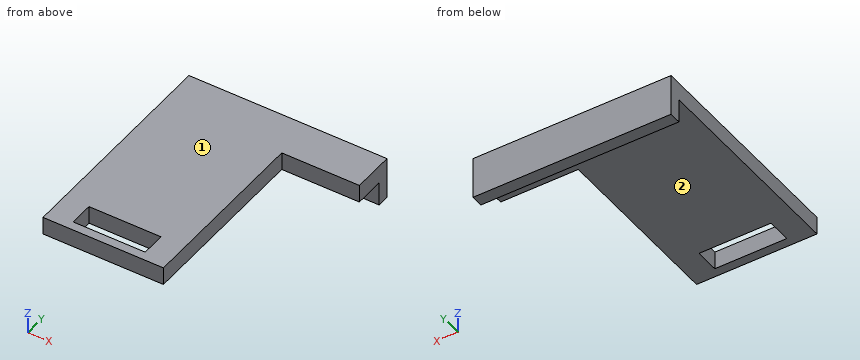
Autodesk Inventor part; units mm, degrees
ref_plane "YZ Plane" through (0, 0, 0) normal (1, 0, 0) x (0, 1, 0)
ref_plane "XZ Plane" through (0, 0, 0) normal (0, 1, 0) x (-1, 0, 0)
ref_plane "XY Plane" through (0, 0, 0) normal (0, 0, 1) x (1, 0, 0)
sketch "Sketch1" plane through (0, 0, 0) normal (0, 0, 1) x (1, 0, 0)
  line L0 (-3.1754, 5) -> (-49.0181, 5)
  line L1 (-3.1754, 40) -> (-3.1754, 5)
  line L2 (-97.8609, 40) -> (-3.1754, 40)
  line L3 (-97.8609, 5) -> (-97.8609, 40)
  line L4 (-52.0181, 5) -> (-97.8609, 5)
  line L5 (-52.0181, 5) -> (-52.0181, 37)
  line L6 (-52.0181, 37) -> (-49.0181, 37)
  line L7 (-49.0181, 37) -> (-49.0181, 5)
  line L8 (-52.0181, 5) -> (-85.0042, 5)
  line L9 (-85.0042, 5) -> (-85.0042, 50)
  line L10 (-85.0042, 50) -> (-52.0181, 50)
  line L11 (-52.0181, 50) -> (-52.0181, 5)
  line L12 (-52.0181, 10.5351) -> (-74.9481, 10.5351) construction
  point P0 (0, 0)
  point P1 (-66.8598, 10.5351)
  dimension "d1" = 45
  dimension "d7" = 45.8427
  dimension "d8" = 22.93
extrude "Extrusion1" add sketch "Sketch1" along normal blind 3 contours L11 L5 L4 L9 L2 | L2 L9 L10 L11
sketch "Sketch2" plane through (0, 0, 0) normal (0, 0, -1) x (-1, 0, 0)
  line L0 (95.2628, 40) -> (95.2628, 0)
  line L1 (5.7735, 40) -> (95.2628, 40)
  line L2 (5.7735, 0) -> (5.7735, 40)
  line L3 (95.2628, 0) -> (5.7735, 0)
  line L4 (52.0181, 5) -> (52.0181, 50)
  line L5 (85.0042, 5) -> (52.0181, 5)
  line L6 (85.0042, 50) -> (85.0042, 5)
  line L7 (52.0181, 50) -> (85.0042, 50)
  line L8 (52.0181, 50) -> (85.0042, 50)
  line L9 (85.0042, 50) -> (85.0042, 40)
  line L10 (85.0042, 40) -> (52.0181, 40)
  line L11 (52.0181, 40) -> (52.0181, 50)
  point P0 (0, 0)
extrude "Extrusion2" add sketch "Sketch2" along normal blind 4 contours L1 L4 L7 L6
sketch "Sketch3" plane through (0, 0, 3) normal (0, 0, 1) x (1, 0, 0)
  line L0 (-80.9481, 10.4777) -> (-68.9481, 10.4777)
  line L1 (-68.9481, 10.4777) -> (-68.9481, 6.4777)
  line L2 (-68.9481, 6.4777) -> (-80.9481, 6.4777)
  line L3 (-80.9481, 6.4777) -> (-80.9481, 10.4777)
  line L4 (-80.9481, 10.4777) -> (-68.9481, 6.4777) construction
  line L5 (-68.9481, 10.4777) -> (-80.9481, 6.4777) construction
  circle A0 centre (-74.9481, 8.4777) radius 2 construction
  circle A1 centre (-71.4481, 8.4777) radius 2 construction
  circle A2 centre (-71.7614, 8.4777) radius 2 construction
  line L6 (-52.0181, 5) -> (-52.0181, 50)
  point P0 (0, 0)
  point P1 (-71.4481, 8.4777)
  dimension "d9" = 12
  dimension "d10" = 4
  dimension "d11" = 4
  dimension "d12" = 3.5
  dimension "d13" = 3.5
  dimension "d23" = 22.93
extrude "Extrusion3" cut sketch "Sketch3" against normal blind 4
sketch "Sketch5" plane through (0, 0, 3) normal (0, 0, 1) x (1, 0, 0)
  line L0 (-80.9481, 6.4777) -> (-80.9481, 10.4777)
  line L1 (-80.9481, 10.4777) -> (-68.9481, 10.4777)
  line L2 (-68.9481, 10.4777) -> (-68.9481, 6.4777)
  line L3 (-68.9481, 6.4777) -> (-80.9481, 6.4777)
  line L4 (-52.0181, 5) -> (-52.0181, 50)
  line L5 (-52.0181, 50) -> (-85.0042, 50)
  line L6 (-85.0042, 50) -> (-85.0042, 5)
  line L7 (-85.0042, 5) -> (-52.0181, 5)
  line L8 (-64.9481, 5) -> (-64.9481, 35)
  line L9 (-64.9481, 35) -> (-52.0181, 35)
  point P0 (0, 0)
  dimension "d39" = 30
  dimension "d40" = 4
extrude "Extrusion5" cut sketch "Sketch5" against normal blind 4 contours L7 L8 L9 L4
chamfer "Chamfer1" [suppressed]
sketch "Sketch6" plane through (0, 0, 3) normal (0, 0, 1) x (1, 0, 0)
  line L0 (-64.9481, 35) -> (-52.0181, 35)
  line L1 (-52.0181, 35) -> (-52.0181, 50)
  line L2 (-52.0181, 50) -> (-85.0042, 50)
  line L3 (-85.0042, 50) -> (-85.0042, 5)
  line L4 (-85.0042, 5) -> (-64.9481, 5)
  line L5 (-64.9481, 5) -> (-64.9481, 35)
  line L6 (-80.9481, 6.4777) -> (-80.9481, 10.4777)
  line L7 (-80.9481, 10.4777) -> (-68.9481, 10.4777)
  line L8 (-68.9481, 10.4777) -> (-68.9481, 6.4777)
  line L9 (-68.9481, 6.4777) -> (-80.9481, 6.4777)
  line L10 (-52.0181, 35) -> (-52.0181, 50)
  line L11 (-85.0042, 50) -> (-52.0181, 50)
  line L12 (-52.0181, 50) -> (-52.0181, 42)
  line L13 (-52.0181, 42) -> (-85.0042, 42)
  line L14 (-85.0042, 42) -> (-85.0042, 50)
  point P0 (0, 0)
  dimension "d44" = 8
extrude "Extrusion6" cut sketch "Sketch6" against normal blind 12.5 contours L13 L3 L2 L1
sketch "Sketch4" plane through (0, 0, 3) normal (0, 0, 1) x (1, 0, 0)
  line L0 (-80.9481, 6.4777) -> (-80.9481, 10.4777)
  line L1 (-80.9481, 10.4777) -> (-68.9481, 10.4777)
  line L2 (-68.9481, 10.4777) -> (-68.9481, 6.4777)
  line L3 (-68.9481, 6.4777) -> (-80.9481, 6.4777)
  line L4 (-52.0181, 5) -> (-52.0181, 50)
  line L5 (-52.0181, 50) -> (-85.0042, 50)
  line L6 (-85.0042, 50) -> (-85.0042, 5)
  line L7 (-85.0042, 5) -> (-52.0181, 5)
  line L8 (-81.0042, 47) -> (-56.0181, 47)
  line L9 (-56.0181, 47) -> (-56.0181, 42)
  line L10 (-56.0181, 42) -> (-81.0042, 42)
  line L11 (-81.0042, 42) -> (-81.0042, 47)
  line L12 (-81.0042, 38) -> (-56.0181, 38)
  line L13 (-56.0181, 38) -> (-56.0181, 33)
  line L14 (-56.0181, 33) -> (-81.0042, 33)
  line L15 (-81.0042, 33) -> (-81.0042, 38)
  line L16 (-81.0042, 29) -> (-56.0181, 29)
  line L17 (-56.0181, 29) -> (-56.0181, 24)
  line L18 (-56.0181, 24) -> (-81.0042, 24)
  line L19 (-81.0042, 24) -> (-81.0042, 29)
  line L20 (-81.0042, 20) -> (-56.0181, 20)
  line L21 (-56.0181, 20) -> (-56.0181, 15)
  line L22 (-56.0181, 15) -> (-81.0042, 15)
  line L23 (-81.0042, 15) -> (-81.0042, 20)
  point P0 (0, 0)
  dimension "d24" = 4
  dimension "d25" = 4
  dimension "d26" = 3
  dimension "d27" = 5
  dimension "d30" = 9
equation "\"d25\" = d24"
properties part number "Aligner Helper v3"
Input: part model. Units: mm. Frame: model coordinates. Face numbers are marked on the shaded views. A direction names the side the tool comes from. Give positions to 0.01 mm unless a question says otherwise; leave off trailing zeros. Loops run counter-clockwise (first coordinate to the right, second up) from the corner with the lowest first, then second, coordinate; pieces in that order, holes last. Notation, with made-up numbers: (41, 21) -> (71, 21) arc R14 ccw to (71, 29) -> close; hole circle Ø4 at (38, 54.5). An arc over 180 degrees is marked (long way). Use a Markdown table: item, result.
Q1. Access query for the marked faces 1 and 2. Directions: +Z, -Z, +X, -X, +Y, -Y. A direction counts if a zero-diameter tool reaches every point of the face in a straight line with its end or side. Return the directions, or none.
Entries:
| item | result |
|---|---|
| face 1 | +Z, +X, -X, +Y, -Y |
| face 2 | -Z, +X, -X, -Y |
Q2. Section query A-A, the plane x = -79. Return the cut outline in (y, z), plus the area to 3 significant figures.
Entries:
| item | result |
|---|---|
| outline | (5, 0) -> (6.48, 0) -> (6.48, 3) -> (5, 3) -> close; (10.48, 0) -> (40, 0) -> (40, -4) -> (42, -4) -> (42, 3) -> (10.48, 3) -> close |
| area | 107 mm² |
Q3. Ray query, probe 1 along Y at (x, z) = (-69.5, 0.5); probe 2 along Z at (x, y) = (-77, 29); probe 3 along X at (y, z) = (28, 2.5). Return the intervals inside material, ascending. Write a range as from..to.
Entries:
| item | result |
|---|---|
| probe 1 | y = 5..6.48, 10.48..42 |
| probe 2 | z = 0..3 |
| probe 3 | x = -85..-64.95 |
Q4. Section query D-D, the plane z = -2.25. Return the cut outline in (x, y).
Entries:
| item | result |
|---|---|
| outline | (-85, 40) -> (-52.02, 40) -> (-52.02, 42) -> (-85, 42) -> close |
Q5. First-contact query: P1, Ø3.5, axis at x = -61.5, z = 1, coming from the -Y side; P2, Ø1, axis at x = -80, z = -3, coming from the -Y side; P3, Ø0.9, axis at y = 8, z = 2, coming from the +X side. Flat tips, straight axial feed; report the tip coordinate or a pass-through.
Entries:
| item | result |
|---|---|
| P1 | stops at y = 35 |
| P2 | stops at y = 40 |
| P3 | stops at x = -64.95 |
Q6. Section query B-B, the plane z = 1.5. Return the cut outline in (x, y), plus the area to 3 significant figures.
Entries:
| item | result |
|---|---|
| outline | (-85, 5) -> (-64.95, 5) -> (-64.95, 35) -> (-52.02, 35) -> (-52.02, 42) -> (-85, 42) -> close; hole (-80.95, 6.48) -> (-68.95, 6.48) -> (-68.95, 10.48) -> (-80.95, 10.48) -> close |
| area | 785 mm² |
Q7. Section query C-C, the plane x = -82.5. Return the cut outline in (y, z).
Entries:
| item | result |
|---|---|
| outline | (5, 0) -> (40, 0) -> (40, -4) -> (42, -4) -> (42, 3) -> (5, 3) -> close |
